For this review, take the finished solid that the model builds, in its own axes (mm). Face numbers are marked on the shaded views. A direction names the side the tool comes from. Coordinates: 2 decimals unless noted, no trailing zeros. Loops run counter-clockwise (first coordinate to the right, second up) from the corner with the lowest first, then second, coordinate; pieces in that order, holes last. Notation, with made-up numbers: (78, 48.25) - (133, 48.25) arc R18 cw to (133, 76.25) - close; hole circle Ø4 at (-23, 5). An arc over 180 degrees is marked (long way). Use one line per item in the form item = value. Start each with the question number.
1. To check wall thickness, follow probe 1 along X at (y, z) = (6.75, 8); probe 2 along X at (y, z) = (0.35, 18); probe 3 along Z at (x, y) = (-80, 0.45). State the ranges of each line that lie inside material, in increasing order.
2. Machinability: for the marked faces 4, 5 and 6, which of the approach directions +Z, -Z, +X, -X, +Y, -Y give a long, thin tool a straight path to every point of the face, cutting with its end or side? Answer none if there is none.
3. Add section D-D on y = 9. Give the boundary of the cut face in (x, z), and give its area (3 significant figures).
4. Add section B-B on y = 3. Give the boundary of the cut face in (x, z).
5. Draft analysis for pull direction Z (two halves, no side actions). For the marked faces 1, 2 and 3, state which applies: +Z half, -Z half, draft (parallel to the pull), parting line (faces both ways), or undercut.
6. For pin 1 Ø6 at (x, z) = (-10, 7) entering from +Y; pin 2 Ø8 at (x, y) = (-25, -0.5) entering from +Z; pin 3 Ø1.5 at (x, z) = (-55.5, 31) entering from -Y, all flat-tipped, find the tip position at first contact; note any pin that passes through.
7. Add section C-C on x = -25.5. Give the boundary of the cut face in (y, z).
8. Add section A-A on x = -80. Give the boundary of the cut face in (y, z), and give its area (3 significant figures).
Autodesk Inventor part; units mm, degrees
ref_plane "YZ Plane" through (0, 0, 0) normal (1, 0, 0) x (0, 1, 0)
ref_plane "XZ Plane" through (0, 0, 0) normal (0, 1, 0) x (-1, 0, 0)
ref_plane "XY Plane" through (0, 0, 0) normal (0, 0, 1) x (1, 0, 0)
sketch "Skizze1" plane through (0, 0, 0) normal (0, 1, 0) x (-1, 0, 0)
  line L0 (0, 0) -> (85, 0)
  line L1 (85, 0) -> (85, 56)
  line L2 (85, 56) -> (0, 56)
  line L3 (0, 56) -> (0, 0)
  dimension "d0" = 85
  dimension "d1" = 56
extrude "Extrusion1" add sketch "Skizze1" along normal blind 1.5
sketch "Skizze2" plane through (0, 1.5, 0) normal (0, 1, 0) x (1, 0, 0)
  line L0 (0, 0) -> (-85, 0)
  line L1 (-86, -17.2) -> (-65, -17.2)
  line L2 (-65, -17.2) -> (-65, -1.2)
  line L3 (-65, -1.2) -> (-86, -1.2)
  line L4 (-86, -1.2) -> (-86, -17.2)
  line L5 (-85, 0) -> (-85, -56)
  dimension "d4" = 21
  dimension "d5" = 16
  dimension "d6" = 1.2
  dimension "d84" = 1
extrude "Extrusion2" add sketch "Skizze2" along normal blind 13.4
sketch "Skizze3" plane through (0, 1.5, 0) normal (0, 1, 0) x (1, 0, 0)
  line L0 (-65, -17.2) -> (-85, -17.2)
  line L1 (-85, -17.2) -> (-85, -56)
  line L2 (-92.5, -23.8) -> (-75.1, -23.8)
  line L3 (-75.1, -23.8) -> (-75.1, -37)
  line L4 (-75.1, -37) -> (-92.5, -37)
  line L5 (-92.5, -37) -> (-92.5, -23.8)
  dimension "d9" = 7.5
  dimension "d10" = 17.4
  dimension "d11" = 13.2
  dimension "d12" = 6.6
extrude "Extrusion3" add sketch "Skizze3" along normal blind 16
sketch "Skizze4" plane through (0, 1.5, 0) normal (0, 1, 0) x (1, 0, 0)
  line L0 (0, 0) -> (-85, 0)
  line L1 (-65, -1.2) -> (-65, -17.2)
  line L2 (-50, 1) -> (-35, 1)
  line L3 (-35, 1) -> (-35, -10.8)
  line L4 (-35, -10.8) -> (-50, -10.8)
  line L5 (-50, -10.8) -> (-50, 1)
  dimension "d15" = 1
  dimension "d16" = 15
  dimension "d17" = 11.8
  dimension "d18" = 15
extrude "Extrusion4" add sketch "Skizze4" along normal blind 5.5
sketch "Skizze5" plane through (0, 1.5, 0) normal (0, 1, 0) x (1, 0, 0)
  line L0 (-85, -37) -> (-85, -56)
  line L1 (-85, -56) -> (0, -56)
  line L2 (-58.5, -44.5) -> (-70.5, -44.5)
  line L3 (-70.5, -44.5) -> (-70.5, -56)
  line L4 (-70.5, -56) -> (-58.5, -56)
  line L5 (-58.5, -56) -> (-58.5, -44.5)
  line L6 (-70.5, -56) -> (-58.5, -56)
  dimension "d21" = 11.5
  dimension "d22" = 12
  dimension "d23" = 14.5
extrude "Extrusion5" add sketch "Skizze5" along normal blind 10
sketch "Skizze6" plane through (-85, 0, 56) normal (0, 0, 1) x (1, 0, 0)
  line L0 (14.5, 11.5) -> (26.5, 11.5)
  circle A0 centre (20.5, 8) radius 3.5
  dimension "d26" = 7
  dimension "d27" = 3.5
extrude "Extrusion6" add sketch "Skizze6" along normal blind 3.5
sketch "Skizze7" plane through (0, 1.5, 0) normal (0, 1, 0) x (1, 0, 0)
  line L0 (-58.5, -44.5) -> (-58.5, -56)
  line L1 (-58.5, -56) -> (0, -56)
  line L2 (-51, -43.5) -> (-41, -43.5)
  line L3 (-41, -43.5) -> (-41, -53.5)
  line L4 (-41, -53.5) -> (-51, -53.5)
  line L5 (-51, -53.5) -> (-51, -43.5)
  dimension "d30" = 10
  dimension "d31" = 10
  dimension "d32" = 2.5
  dimension "d33" = 7.5
extrude "Extrusion7" add sketch "Skizze7" along normal blind 14.5
sketch "Skizze8" plane through (-51, 1.5, 53.5) normal (0, 0, 1) x (1, 0, 0)
  line L0 (0, 14.5) -> (10, 14.5)
  circle A0 centre (5, 10.5) radius 4
  point P0 (51, -1.5)
  dimension "d36" = 8
  dimension "d37" = 0
extrude "Extrusion8" add sketch "Skizze8" along normal blind 9
sketch "Skizze9" plane through (0, 1.5, 0) normal (0, 1, 0) x (1, 0, 0)
  line L0 (-58.5, -56) -> (0, -56)
  line L1 (0, -56) -> (0, 0)
  line L2 (-1, -55) -> (-33.7, -55)
  line L3 (-33.7, -55) -> (-33.7, -50)
  line L4 (-33.7, -50) -> (-1, -50)
  line L5 (-1, -50) -> (-1, -55)
  dimension "d40" = 32.7
  dimension "d41" = 5
  dimension "d42" = 1
  dimension "d43" = 1
extrude "Extrusion9" add sketch "Skizze9" along normal blind 2.5
sketch "Skizze10" plane through (0, 4, 0) normal (0, 1, 0) x (1, 0, 0)
  line L0 (-33.7, -55) -> (-1, -55)
  line L1 (-1, -55) -> (-1, -50)
  line L2 (-1, -50) -> (-33.7, -50)
  line L3 (-33.7, -50) -> (-33.7, -55)
  line L4 (-32.7, -51) -> (-2, -51)
  line L5 (-2, -51) -> (-2, -54)
  line L6 (-2, -54) -> (-32.7, -54)
  line L7 (-32.7, -54) -> (-32.7, -51)
  point P0 (0, 0)
  dimension "d50" = 1
  dimension "d51" = 1
  dimension "d52" = 1
  dimension "d53" = 1
extrude "Extrusion10" add sketch "Skizze10" along normal blind 6 contours L4 L5 L6 L7
sketch "Skizze11" plane through (0, 1.5, 0) normal (0, 1, 0) x (1, 0, 0)
  line L0 (0, -56) -> (0, 0)
  line L1 (0, 0) -> (-35, 0)
  line L2 (1, -4) -> (-4.6, -4)
  line L3 (-4.6, -4) -> (-4.6, -11.5)
  line L4 (-4.6, -11.5) -> (1, -11.5)
  line L5 (1, -11.5) -> (1, -4)
  dimension "d56" = 1
  dimension "d57" = 7.5
  dimension "d58" = 5.6
  dimension "d59" = 4
extrude "Extrusion11" add sketch "Skizze11" along normal blind 3
sketch "Skizze12" plane through (0, 0, 0) normal (0, -1, 0) x (1, 0, 0)
  line L0 (0, 0) -> (-85, 0)
  line L1 (0, 56) -> (0, 0)
  line L2 (-1, 43.5) -> (-18, 43.5)
  line L3 (-18, 43.5) -> (-18, 15.5)
  line L4 (-18, 15.5) -> (-1, 15.5)
  line L5 (-1, 15.5) -> (-1, 43.5)
  dimension "d62" = 15.5
  dimension "d63" = 17
  dimension "d64" = 28
  dimension "d65" = 1
extrude "Extrusion12" add sketch "Skizze12" along normal blind 0.5
sketch "Skizze13" plane through (0, -0.5, 0) normal (0, -1, 0) x (1, 0, 0)
  line L0 (-1, 43.5) -> (-18, 43.5)
  line L1 (-18, 43.5) -> (-18, 15.5)
  line L2 (-18, 15.5) -> (-1, 15.5)
  line L3 (-1, 15.5) -> (-1, 43.5)
  line L4 (-15, 42.5) -> (-1, 42.5)
  line L5 (-1, 42.5) -> (-1, 18.5)
  line L6 (-1, 18.5) -> (-15, 18.5)
  line L7 (-15, 18.5) -> (-15, 42.5)
  line L8 (-15, 37.5) -> (-10, 42.5)
  line L9 (-15, 37.5) -> (-7.9289, 37.5) construction
  point P0 (0, 0)
  dimension "d69" = 24
  dimension "d70" = 3
  dimension "d71" = 3
  dimension "d72" = 45
  dimension "d73" = 19
extrude "Extrusion13" add sketch "Skizze13" along normal blind 2 contours L3 L4 L7 L6 L2 L1 L0 | L8 L7 L4
sketch "Skizze14" plane through (0, 1.5, 0) normal (0, 1, 0) x (1, 0, 0)
  line L0 (0, 0) -> (-35, 0)
  line L1 (-85, -37) -> (-85, -56)
  line L2 (-85, -56) -> (-70.5, -56)
  line L3 (0, -56) -> (0, -11.5)
  circle A0 centre (-25.5, -18) radius 1.45
  circle A1 centre (-80, -43.5) radius 1.45
  dimension "d76" = 2.9
  dimension "d77" = 25.5
  dimension "d78" = 18
  dimension "d79" = 2.9
  dimension "d80" = 5
  dimension "d81" = 12.5
extrude "Extrusion14" cut sketch "Skizze14" against normal through all
properties part number "PCB"
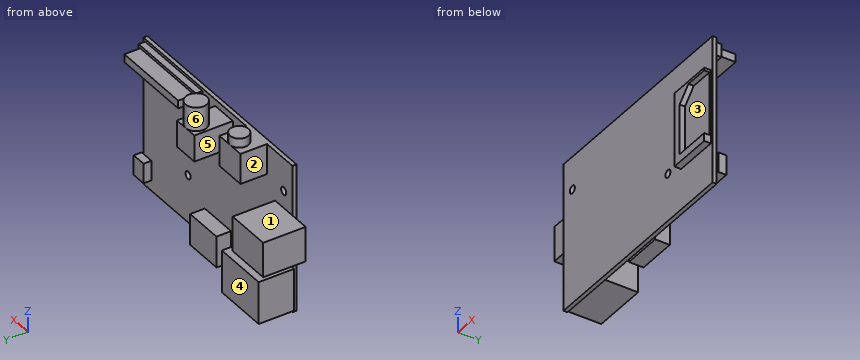
Conclusion:
q1.probe_1 = -86 to -65, -50 to -35
q1.probe_2 = -85 to -26.95, -24.05 to 0
q1.probe_3 = 0 to 42.05, 44.95 to 56
q2.face_4 = -Z, +X, -X, +Y
q2.face_5 = +Z, -Z, +Y
q2.face_6 = +Z
q3.outline = (-92.5, 23.8) - (-75.1, 23.8) - (-75.1, 37) - (-92.5, 37) - close; (-86, 1.2) - (-65, 1.2) - (-65, 17.2) - (-86, 17.2) - close; (-70.5, 44.5) - (-58.5, 44.5) - (-58.5, 56) - (-61.15, 56) - (-61.15, 59.5) - (-67.85, 59.5) - (-67.85, 56) - (-70.5, 56) - close; (-51, 43.5) - (-41, 43.5) - (-41, 53.5) - (-43.35, 53.5) - (-43.35, 62.5) - (-48.65, 62.5) - (-48.65, 53.5) - (-51, 53.5) - close; (-32.7, 51) - (-2, 51) - (-2, 54) - (-32.7, 54) - close
q3.area = 967 mm^2
q4.outline = (-92.5, 23.8) - (-75.1, 23.8) - (-75.1, 37) - (-92.5, 37) - close; (-86, 1.2) - (-65, 1.2) - (-65, 17.2) - (-86, 17.2) - close; (-70.5, 44.5) - (-58.5, 44.5) - (-58.5, 56) - (-70.5, 56) - close; (-51, 43.5) - (-41, 43.5) - (-41, 53.5) - (-51, 53.5) - close; (-50, -1) - (-35, -1) - (-35, 10.8) - (-50, 10.8) - close; (-33.7, 50) - (-1, 50) - (-1, 55) - (-33.7, 55) - close; (-4.6, 4) - (1, 4) - (1, 11.5) - (-4.6, 11.5) - close
q5.face_1 = +Z half
q5.face_2 = draft
q5.face_3 = undercut
q6.pin_1 = 1.5
q6.pin_2 = 56
q6.pin_3 = 0
q7.outline = (0, 0) - (1.5, 0) - (1.5, 16.55) - (0, 16.55) - close; (0, 19.45) - (1.5, 19.45) - (1.5, 50) - (4, 50) - (4, 51) - (10, 51) - (10, 54) - (4, 54) - (4, 55) - (1.5, 55) - (1.5, 56) - (0, 56) - close
q8.outline = (0, 0) - (1.5, 0) - (1.5, 1.2) - (14.9, 1.2) - (14.9, 17.2) - (1.5, 17.2) - (1.5, 23.8) - (17.5, 23.8) - (17.5, 37) - (1.5, 37) - (1.5, 42.05) - (0, 42.05) - close; (0, 44.95) - (1.5, 44.95) - (1.5, 56) - (0, 56) - close
q8.area = 505 mm^2
